Work out the finished part from the listing and answer in its coordinate system (mm). Face numbers are marked on the shaded views. Give positions to 0.01 mm unless a question says otherwise; leave off trailing zeros. Loops run counter-clockwise (first coordinate to the right, second up) from the corner with the lowest first, then second, coordinate; pieces in that order, holes last. Notation, with made-up numbers: (-10.5, -31) - (-1.5, -31) arc R22 ccw to (-1.5, -14) - close; hole circle Ø6 at (60.25, 20). An arc over 180 degrees is marked (long way). One line per item, written item: value.
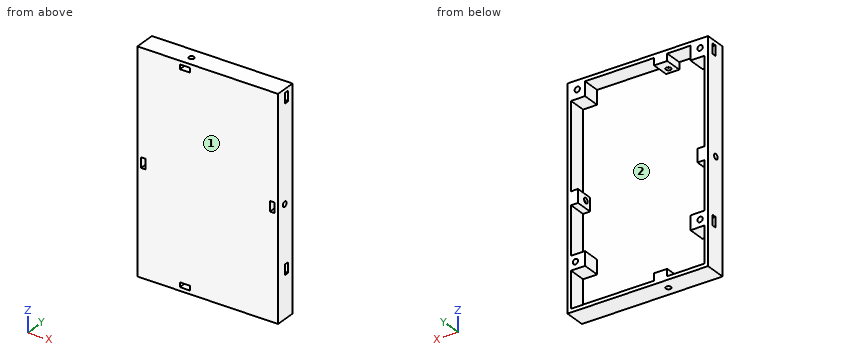
Autodesk Inventor part; units mm, degrees
ref_plane "YZ Plane" through (0, 0, 0) normal (1, 0, 0) x (0, 1, 0)
ref_plane "XZ Plane" through (0, 0, 0) normal (0, 1, 0) x (-1, 0, 0)
ref_plane "XY Plane" through (0, 0, 0) normal (0, 0, 1) x (1, 0, 0)
sketch "Sketch1" plane through (0, 0, 0) normal (0, 1, 0) x (-1, 0, 0)
  line L0 (0, 0) -> (80, 0)
  line L1 (80, 0) -> (80, -124)
  line L2 (80, -124) -> (0, -124)
  line L3 (0, -124) -> (0, 0)
  dimension "d0" = 80
  dimension "d1" = 124
extrude "Extrusion1" add sketch "Sketch1" along normal blind 12
sketch "Sketch2" plane through (0, 12, 0) normal (0, 1, 0) x (1, 0, 0)
  line L0 (0, 0) -> (0, 124)
  line L1 (0, 124) -> (-2, 124)
  line L2 (0, 124) -> (-80, 124)
  line L3 (-2, 124) -> (-2, 122)
  line L4 (-2, 122) -> (-78, 122)
  line L5 (-78, 122) -> (-78, 2)
  line L6 (-78, 2) -> (-2, 2)
  line L7 (-2, 2) -> (-2, 122)
  dimension "d4" = 2
  dimension "d5" = 2
  dimension "d6" = 270
  dimension "d7" = 76
  dimension "d8" = 120
extrude "Extrusion2" cut sketch "Sketch2" against normal blind 10
sketch "Sketch5" plane through (0, 2, 0) normal (0, 1, 0) x (1, 0, 0)
  line L0 (-2, 2) -> (-78, 2)
  line L1 (-2, 2) -> (-10, 2)
  line L2 (-10, 2) -> (-10, 10)
  line L3 (-10, 10) -> (-2, 10)
  line L4 (-2, 10) -> (-2, 2)
  line L5 (-2, 2) -> (-4.5, 2)
  line L6 (-4.5, 2) -> (-4.5, 5)
  line L7 (-78, 2) -> (-70, 2)
  line L8 (-70, 2) -> (-70, 10)
  line L9 (-70, 10) -> (-78, 10)
  line L10 (-78, 10) -> (-78, 2)
  line L11 (-2, 2) -> (-78, 2)
  line L12 (-78, 2) -> (-78, 101.45)
  line L13 (-78, 2) -> (21.45, 2) construction
  line L14 (-2, 122) -> (-2, 2)
  line L15 (-2, 2) -> (-2, 101.45)
  line L16 (-2, 2) -> (97.45, 2) construction
  line L17 (-78, 101.45) -> (-70, 101.45)
  line L18 (-70, 101.45) -> (-70, 93.45)
  line L19 (-70, 93.45) -> (-78, 93.45)
  line L20 (-78, 93.45) -> (-78, 101.45)
  line L21 (-2, 101.45) -> (-10, 101.45)
  line L22 (-10, 101.45) -> (-10, 93.45)
  line L23 (-10, 93.45) -> (-2, 93.45)
  line L24 (-2, 93.45) -> (-2, 101.45)
  point P0 (0, 0)
  dimension "d31" = 8
  dimension "d32" = 8
  dimension "d34" = 2.5
  dimension "d35" = 3
  dimension "d36" = 8
  dimension "d37" = 8
  dimension "d83" = 99.45
  dimension "d84" = 90
  dimension "d85" = 99.45
  dimension "d86" = 90
  dimension "d87" = 8
  dimension "d88" = 8
  dimension "d89" = 8
  dimension "d90" = 8
extrude "Extrusion8" add sketch "Sketch5" along normal blind 10
sketch "Sketch9" plane through (0, 12, 0) normal (0, 1, 0) x (1, 0, 0)
  circle A0 centre (-5.5701, 5) radius 1.5
  circle A1 centre (-75.5, 5) radius 1.5
  circle A2 centre (-4.5, 97.45) radius 1.5
  circle A3 centre (-75.5, 97.45) radius 1.5
  line L0 (-70, 101.45) -> (-78, 101.45)
  line L1 (-78, 10) -> (-78, 93.45)
  line L2 (-10, 2) -> (-70, 2)
  line L3 (-10, 10) -> (-10, 2)
  line L4 (-10, 93.45) -> (-2, 93.45)
  line L5 (-2, 93.45) -> (-2, 10)
  point P0 (0, 0)
  dimension "d93" = 4
  dimension "d94" = 2.5
  dimension "d95" = 3
  dimension "d96" = 2.5
  dimension "d97" = 3
  dimension "d98" = 4.4299
  dimension "d99" = 3
  dimension "d100" = 4
  dimension "d101" = 2.5
extrude "Extrusion9" cut sketch "Sketch9" against normal blind 10
sketch "Sketch11" plane through (0, 0, -124) normal (0, 0, -1) x (-1, 0, 0)
  line L0 (80, 0) -> (80, 12)
  line L1 (80, 0) -> (53, 0)
  line L2 (0, 0) -> (80, 0)
  line L3 (53, 0) -> (53, 5.5)
  circle A0 centre (53, 5.5) radius 1.5
  dimension "d107" = 27
  dimension "d108" = 5.5
  dimension "d109" = 3
sketch "Sketch12" plane through (0, 0, 0) normal (1, 0, 0) x (0, 0, -1)
  line L0 (0, 0) -> (0, 12)
  line L1 (0, 0) -> (0, 5.85)
  line L2 (0, 5.85) -> (2.125, 5.85)
  line L3 (2.125, 5.85) -> (7.875, 5.85)
  line L4 (7.875, 5.85) -> (7.875, 8.45)
  line L5 (7.875, 8.45) -> (2.125, 8.45)
  line L6 (2.125, 8.45) -> (2.125, 5.85)
  line L7 (124, 0) -> (0, 0)
  line L8 (7.875, 5.85) -> (94.575, 5.85)
  line L9 (10, 12) -> (10, 2)
  line L10 (7.875, 5.85) -> (94.575, 5.85) construction
  line L11 (94.575, 5.85) -> (100.325, 5.85)
  line L12 (100.325, 5.85) -> (100.325, 8.45)
  line L13 (100.325, 8.45) -> (94.575, 8.45)
  line L14 (94.575, 8.45) -> (94.575, 5.85)
  dimension "d112" = 5.85
  dimension "d113" = 2.125
  dimension "d114" = 5.75
  dimension "d115" = 2.6
  dimension "d122" = 86.7
  dimension "d123" = 0
  dimension "d124" = 5.75
  dimension "d125" = 2.6
extrude "Extrusion11" cut sketch "Sketch12" against normal blind 8
sketch "Sketch13" plane through (-80, 0, -124) normal (-1, 0, 0) x (0, 0, 1)
  line L0 (124, 0) -> (124, 5.85)
  line L1 (124, 0) -> (124, 12)
  line L2 (124, 5.85) -> (121.875, 5.85)
  line L3 (121.875, 5.85) -> (116.125, 5.85)
  line L4 (116.125, 5.85) -> (116.125, 8.45)
  line L5 (116.125, 8.45) -> (121.875, 8.45)
  line L6 (121.875, 8.45) -> (121.875, 5.85)
  line L7 (116.125, 5.85) -> (29.425, 5.85)
  line L8 (114, 2) -> (114, 12)
  line L9 (116.125, 5.85) -> (202.825, 5.85) construction
  line L10 (29.425, 5.85) -> (23.675, 5.85)
  line L11 (23.675, 5.85) -> (23.675, 8.45)
  line L12 (23.675, 8.45) -> (29.425, 8.45)
  line L13 (29.425, 8.45) -> (29.425, 5.85)
  dimension "d126" = 5.85
  dimension "d127" = 2.125
  dimension "d128" = 5.75
  dimension "d129" = 2.6
  dimension "d130" = 86.7
  dimension "d131" = 180
  dimension "d132" = 5.75
  dimension "d181" = 2.6
extrude "Extrusion12" cut sketch "Sketch13" against normal blind 8
sketch "Sketch14" plane through (0, 0, 0) normal (1, 0, 0) x (0, 0, -1)
  line L0 (0, 0) -> (124, 0)
  line L1 (0, 0) -> (62, 0)
  line L2 (62, 0) -> (62, 5.5)
  circle A0 centre (62, 5.5) radius 1.5
  line L3 (0, 0) -> (0, 12)
  dimension "d135" = 5.5
  dimension "d136" = 3
  dimension "d139" = 62
sketch "Sketch15" plane through (0, 2, 0) normal (0, 1, 0) x (1, 0, 0)
  line L0 (-80, 0) -> (0, 0)
  line L1 (-80, 0) -> (-56.75, 0)
  line L2 (-56.75, 0) -> (-56.75, 2)
  line L3 (-10, 2) -> (-70, 2)
  line L4 (-56.75, 2) -> (-49.25, 2)
  line L5 (-49.25, 2) -> (-49.25, 6)
  line L6 (-49.25, 6) -> (-56.75, 6)
  line L7 (-56.75, 6) -> (-56.75, 2)
  line L8 (0, 124) -> (-80, 124)
  line L9 (-80, 124) -> (-56.75, 124)
  line L10 (-56.75, 124) -> (-56.75, 122)
  line L11 (-78, 122) -> (-2, 122)
  line L12 (-56.75, 122) -> (-49.25, 122)
  line L13 (-49.25, 122) -> (-49.25, 118)
  line L14 (-49.25, 118) -> (-56.75, 118)
  line L15 (-56.75, 118) -> (-56.75, 122)
  line L16 (0, 0) -> (0, 58.75)
  line L17 (0, 0) -> (0, 124)
  line L18 (0, 58.75) -> (-2, 58.75)
  line L19 (-2, 93.45) -> (-2, 10)
  line L20 (-2, 58.75) -> (-6, 58.75)
  line L21 (-6, 58.75) -> (-6, 66.25)
  line L22 (-6, 66.25) -> (-2, 66.25)
  line L23 (-2, 66.25) -> (-2, 58.75)
  line L24 (-80, 0) -> (-80, 58.75)
  line L25 (-80, 124) -> (-80, 0)
  line L26 (-80, 58.75) -> (-78, 58.75)
  line L27 (-78, 10) -> (-78, 93.45)
  line L28 (-78, 58.75) -> (-74, 58.75)
  line L29 (-74, 58.75) -> (-74, 66.25)
  line L30 (-74, 66.25) -> (-78, 66.25)
  line L31 (-78, 66.25) -> (-78, 58.75)
  dimension "d140" = 23.25
  dimension "d141" = 7.5
  dimension "d142" = 4
  dimension "d143" = 23.25
  dimension "d144" = 7.5
  dimension "d145" = 4
  dimension "d146" = 58.75
  dimension "d147" = 4
  dimension "d148" = 7.5
  dimension "d149" = 58.75
  dimension "d150" = 4
  dimension "d151" = 7.5
extrude "Extrusion14" add sketch "Sketch15" along normal blind 10 contours L7 L6 L5 L3 | L20 L21 L22 L19 | L11 L13 L14 L15 | L27 L30 L29 L28
extrude "Extrusion15" cut sketch "Sketch11" against normal blind 124
extrude "Extrusion16" cut sketch "Sketch14" against normal blind 82
sketch "Sketch16" plane through (0, 0, 0) normal (0, -1, 0) x (1, 0, 0)
  line L0 (-80, 0) -> (0, 0)
  line L1 (-80, 0) -> (-55.875, 0)
  line L2 (-55.875, 0) -> (-55.875, -2)
  line L3 (-55.875, -2) -> (-50.125, -2)
  line L4 (-50.125, -2) -> (-50.125, -4.6)
  line L5 (-50.125, -4.6) -> (-55.875, -4.6)
  line L6 (-55.875, -4.6) -> (-55.875, -2)
  line L7 (0, -124) -> (-80, -124)
  line L8 (-80, -124) -> (-55.875, -124)
  line L9 (-55.875, -124) -> (-55.875, -122)
  line L10 (-55.875, -122) -> (-50.125, -122)
  line L11 (-50.125, -122) -> (-50.125, -119.4)
  line L12 (-50.125, -119.4) -> (-55.875, -119.4)
  line L13 (-55.875, -119.4) -> (-55.875, -122)
  line L14 (-80, 0) -> (-80, -59.125)
  line L15 (-80, 0) -> (-80, -124)
  line L16 (-80, 0) -> (-20.875, 0) construction
  line L17 (-80, -59.125) -> (-78, -59.125)
  line L18 (-74, -60.5) -> (-74, -63.5)
  line L19 (-78, -59.125) -> (-75.4, -59.125)
  line L20 (-75.4, -59.125) -> (-75.4, -64.875)
  line L21 (-75.4, -64.875) -> (-78, -64.875)
  line L22 (-78, -64.875) -> (-78, -59.125)
  line L23 (0, 0) -> (0, -59.125)
  line L24 (-2, -58.75) -> (-2, -10)
  line L25 (0, 0) -> (59.125, 0) construction
  line L26 (0, -59.125) -> (-2, -59.125)
  line L27 (0, -63.5) -> (-6, -63.5)
  line L28 (-2, -59.125) -> (-4.6, -59.125)
  line L29 (-4.6, -59.125) -> (-4.6, -64.875)
  line L30 (-4.6, -64.875) -> (-2, -64.875)
  line L31 (-2, -64.875) -> (-2, -59.125)
  dimension "d158" = 24.125
  dimension "d162" = 2
  dimension "d163" = 5.75
  dimension "d164" = 2.6
  dimension "d165" = 24.125
  dimension "d166" = 2
  dimension "d167" = 5.75
  dimension "d168" = 2.6
  dimension "d169" = 59.125
  dimension "d170" = 90
  dimension "d171" = 2
  dimension "d172" = 2.6
  dimension "d173" = 5.75
  dimension "d174" = 59.125
  dimension "d175" = 90
  dimension "d176" = 2
  dimension "d177" = 2.6
  dimension "d178" = 5.75
extrude "Extrusion17" cut sketch "Sketch16" against normal blind 8.5
properties part number "Case_Top"
1. Find the intervals of material crossed by line 1 along X through (y, z) = (9.25, -5); line 2 along X through (y, z) = (11.25, -91.5); line 3 along Z through (x, y) = (-72.5, 9.5), in increasing order.
Output:
line 1: x = -80 to -77, -74 to -70, -56.75 to -49.25, -10 to -7.07, -4.07 to 0
line 2: x = -80 to -78, -2 to 0
line 3: z = -124 to -122, -101.45 to -93.45, -10 to 0
2. Section D-D (x = -45) is taken. Write down the section's boundary in (y, z).
Output:
outline: (0, -124) - (12, -124) - (12, -122) - (2, -122) - (2, -2) - (12, -2) - (12, 0) - (0, 0) - close
3. Section A-A (x = -53) is taken. Count the separate pieces of the cut face and the enclosed holes in it, and give its area (3 significant figures).
Output:
separate pieces: 5
enclosed holes: 0
area: 303 mm²
4. A flat-ended cylindrical pin translates along its axis: pin 1 Ø3 at (x, z) = (-48.5, -96.5) entering from +Y. Find the tip coordinate at first contact, or state that the pin passes through.
Output:
pin 1: stops at y = 2
5. The mould has two halves that part along Z. Classify the marked faces 1 and 2: released by +Z, released by -Z, zero draft, split by the parting line, or undercut.
Output:
face 1: zero draft
face 2: undercut
